```python
from build123d import *

# Parameters (mm, degrees)
SKETCH_1_R          = 50
EXTRUDE_1_DEPTH     = 2
SKETCH_2_R          = 50
SKETCH_2_R_2        = 48
EXTRUDE_2_DEPTH     = 3
SKETCH_3_R          = 1
CUT_EXTRUDE_1_DEPTH = 20
FILLET_1_SIZE       = 2


with BuildPart() as part:
    # 草图1 → 凸台-拉伸1 (new body)
    with BuildSketch(Plane(origin=(0, 0, 0), x_dir=(1, 0, 0), z_dir=(0, 1, 0))):
        with Locations(Location((0, 0, 0), (0, 0, 270))):
            Circle(SKETCH_1_R)
    extrude(amount=EXTRUDE_1_DEPTH)

    # 草图2 → 凸台-拉伸2 (add)
    with BuildSketch(Plane(origin=(0, 2, 0), x_dir=(1, 0, 0), z_dir=(0, 1, 0))):
        with Locations(Location((0, 0, 0), (0, 0, 270))):
            Circle(SKETCH_2_R)
        with Locations(Location((0, 0, 0), (0, 0, 270))):
            Circle(SKETCH_2_R_2, mode=Mode.SUBTRACT)
    extrude(amount=EXTRUDE_2_DEPTH)

    # 草图3 → 切除-拉伸1 (cut)
    with BuildSketch(Plane.XZ):
        with Locations(Location((0, 41.598526054, 0), (0, 0, 270))):
            Circle(SKETCH_3_R)
        with Locations(Location((-35.940054257, -20.651473946, 0), (0, 0, 270))):
            Circle(SKETCH_3_R)
        with Locations(Location((35.940054257, -20.651473946, 0), (0, 0, 270))):
            Circle(SKETCH_3_R)
    extrude(amount=-CUT_EXTRUDE_1_DEPTH, mode=Mode.SUBTRACT)

    # 圆角1
    # a fillet whose section is not a circle: 2 mm, written as the material it takes off along each edge
    with BuildSketch(Plane(origin=(0, 0, 41.598526054), x_dir=(0, 0, -1), z_dir=(-1, 0, 0))) as fillet_1_piece_1:
        with BuildLine():
            Bezier((1 + FILLET_1_SIZE, 0), (1, 0), (1, -FILLET_1_SIZE), weights=[1, 0.141421356, 1])
            Line((1, -FILLET_1_SIZE), (1, 0))
            Line((1, 0), (1 + FILLET_1_SIZE, 0))
        make_face()
    revolve(axis=Axis((0, 0, 41.598526054), (0, -1, 0)), mode=Mode.SUBTRACT)
    with BuildSketch(Plane(origin=(-35.940054257, 0, -20.651473946), x_dir=(0, 0, -1), z_dir=(-1, 0, 0))) as fillet_1_piece_2:
        with BuildLine():
            Bezier((1 + FILLET_1_SIZE, 0), (1, 0), (1, -FILLET_1_SIZE), weights=[1, 0.141421356, 1])
            Line((1, -FILLET_1_SIZE), (1, 0))
            Line((1, 0), (1 + FILLET_1_SIZE, 0))
        make_face()
    revolve(axis=Axis((-35.940054257, 0, -20.651473946), (0, -1, 0)), mode=Mode.SUBTRACT)
    with BuildSketch(Plane(origin=(35.940054257, 0, -20.651473946), x_dir=(0, 0, -1), z_dir=(-1, 0, 0))) as fillet_1_piece_3:
        with BuildLine():
            Bezier((1 + FILLET_1_SIZE, 0), (1, 0), (1, -FILLET_1_SIZE), weights=[1, 0.141421356, 1])
            Line((1, -FILLET_1_SIZE), (1, 0))
            Line((1, 0), (1 + FILLET_1_SIZE, 0))
        make_face()
    revolve(axis=Axis((35.940054257, 0, -20.651473946), (0, -1, 0)), mode=Mode.SUBTRACT)


solid = part.part
```
Input: part model. Units: mm. Frame: model coordinates. A direction names the side the tool comes from. Round coordinates to 2 decimals unless told otherwise and drop trailing zeros. Loops run counter-clockwise (first coordinate to the right, second up) from the corner with the lowest first, then second, coordinate; pieces in that order, holes last. Notation, with made-up numbers: M 30.5,24.25 L 40.5,24.25 A31 ccw 40.5,63.25 Z; hole C -39,17.5 d9. An arc over 180 degrees is marked long. Answer in a Markdown table with one row per item. Add a question column.
1. Mould query, pull axis X, two halves, no side actions, for faces 1 (the face through (15.02, 2.46, 47.69)), 2 (the face through (1, 0, -1)), 3 (the face through (14.418, 3.479, 45.783)). Classes: released by +X, released by -X, zero draft, split by the parting line, or undercut.
2. Section A-A (x = 6). Output: boundary loops of the cut face in (y, z).
3. Section C-C (y = 3.6). Output: boundary loops of the cut face in (x, z).
4. Ray query, probe 1 along X at (y, z) = (4, 0); probe 2 along Y at (x, z) = (17, 13.5); probe 3 along X at (y, z) = (2.35, -35). Return the intervals inside material, ascending.
5. Section B-B (z = 0). Output: boundary loops of the cut face in (x, y).
6. Set-up query: faces 4 (the face through (19, 5, -45)), 5 (the face through (1, 2, -1)). Return all of +Z, -Z, +X, -X, +Y, -Y with unobstructed straight access to the full face (end or side cutting, diameter ignored); none if empty.
7. Contact query for a flat-ended pin moving along its axis: pin 1 (8 mm diameter, centred on x = -11.5, z = 32.5, fed in from +Y). Output: stop coordinate, or through.
Values follow:
| question | item | result |
|---|---|---|
| 1 | face 1 | split by the parting line |
| 1 | face 2 | zero draft |
| 1 | face 3 | undercut |
| 2 | outline | M 0,-49.64 L 5,-49.64 L 5,-47.62 L 2,-47.62 L 2,47.62 L 5,47.62 L 5,49.64 L 0,49.64 Z |
| 3 | outline | C 0,0 d100; hole C 0,0 d96 |
| 4 | probe 1 | -50 to -48, 48 to 50 |
| 4 | probe 2 | 0 to 2 |
| 4 | probe 3 | -35.71 to -32.85, 32.85 to 35.71 |
| 5 | outline | M -50,0 L 50,0 L 50,5 L 48,5 L 48,2 L -48,2 L -48,5 L -50,5 Z |
| 6 | face 4 | +Z, -Z, +X, -X, +Y |
| 6 | face 5 | +Y |
| 7 | pin 1 | y = 2 |
